Geometry: final body of the model. Coordinates: model frame, mm. A direction names the side the tool comes from. Coordinates: 2 decimals unless noted, no trailing zeros. Order: outer loops, then holes, each group sorted by start corner. A loop starts at its lowest first (then second) coordinate and runs counter-clockwise, first axis right, second up. Notation, with made-up numbers: M 8,78.5 L 12,78.5 A14 ccw 12,85.5 Z; hole C 70,46 d4. An arc over 180 degrees is marked long. One line per question, with ' | ' between items.
from build123d import *


with BuildPart() as part:
    # Sketch → Revolution (revolve)
    with BuildSketch(Plane.XZ):
        Polygon((3, 35), (7, 35), (10, 5), (10, 0), (0, 0), (0, 1), (3, 1), align=None)
    revolution = revolve(axis=Axis((0, 0, 0), (0, 0, 1)))

    # Mirrored: Revolution across Sketch H_Axis
    add(revolution.mirror(Plane(origin=(0, 0, 0), x_dir=(0, -1, 0), z_dir=(0, 0, 1))))


solid = part.part
1. Access query for faces 1 (the face through (-1, -3, -35)), 2 (the face through (0, 0, -1)), 3 (the face through (-3, 0, 18)). Directions: +Z, -Z, +X, -X, +Y, -Y. A direction counts if a zero-diameter tool reaches every point of the face in a straight line with its end or side. Return the directions, or none.
Response values:
face 1: -Z, +X, -X, +Y, -Y | face 2: -Z | face 3: +Z
2. Section B-B, the plane z = 14.5. Output: boundary loops of the cut face in (x, y).
Response values:
outline: C 0,0 d18.1; hole C 0,0 d6
3. Draft query along X for faces 4 (the face through (8.128, 2.559, -19.79)), 5 (the face through (0, 0, 1)), 6 (the face through (-1, -3, 35)). Return one class per face: pulls with the +X half, pulls with the -X half, needs draft (parallel to the pull), parting line crosses it, or undercut.
Response values:
face 4: parting line crosses it | face 5: undercut | face 6: needs draft
4. Material intervals for line 1 (Z direction, x = -0.25, y = 2.25); line 2 (Y direction, x = 0, z = -19); line 3 (Y direction, x = 0, z = 12), sorted ascending. Write a range as [from, to].
Response values:
line 1: z = [-1, 1] | line 2: y = [-8.6, -3], [3, 8.6] | line 3: y = [-9.3, -3], [3, 9.3]
5. Section A-A, the plane x = 0. Output: boundary loops of the cut face in (y, z), and give its area (3 significant figures).
Response values:
outline: M -10,-5 L -7,-35 L -3,-35 L -3,-1 L 3,-1 L 3,-35 L 7,-35 L 10,-5 L 10,5 L 7,35 L 3,35 L 3,1 L -3,1 L -3,35 L -7,35 L -10,5 Z | area: 812 mm^2
6. Section D-D, the plane z = -23. Output: boundary loops of the cut face in (x, y).
Response values:
outline: C 0,0 d16.4; hole C 0,0 d6
7. Pin query (flat end, axial travel): P1, Ø6, axis at x = -1.5, z = 21, coming from the -Y side; P2, Ø2, axis at y = 2, z = -14, coming from the -X side; P3, Ø8, axis at x = -1.5, z = -22.5, coming from the +Y side. Return the tip coordinate at first contact, or that it passes through.
Response values:
P1: stops at y = -8.67 | P2: stops at x = -9.08 | P3: stops at y = 8.63
